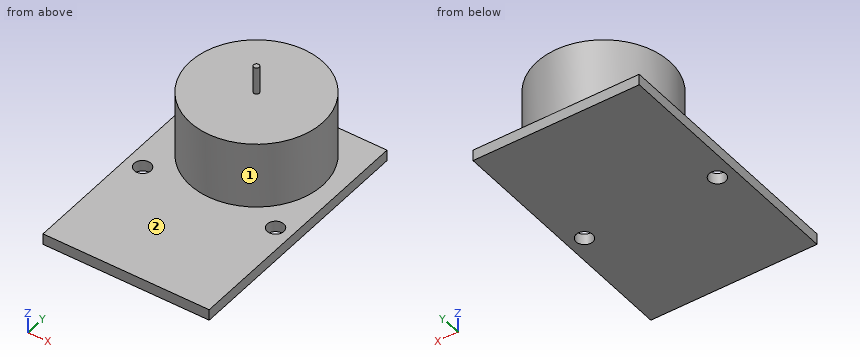
```python
from build123d import *

# Parameters (mm, degrees)
SKETCH_1_W          = 30
SKETCH_1_H          = 45
EXTRUDE_1_DEPTH     = 2
SKETCH_2_R          = 12
EXTRUDE_2_DEPTH     = 12
CUT_EXTRUDE_1_REACH = 31.585
SKETCH_3_R          = 1.5
SKETCH_5_R          = 0.5
EXTRUDE_3_DEPTH     = 5


with BuildPart() as part:
    # 草图1 → 凸台-拉伸1 (new body)
    with BuildSketch(Plane.XY):
        Rectangle(SKETCH_1_W, SKETCH_1_H)
    extrude(amount=-EXTRUDE_1_DEPTH)

    # 草图2 → 凸台-拉伸2 (add)
    with BuildSketch(Plane.XY):
        with Locations(Location((0, 10.5, 0), (0, 0, 90))):
            Circle(SKETCH_2_R)
    extrude(amount=EXTRUDE_2_DEPTH)

    # 草图3 → 切除-拉伸1 (cut, up to next)
    with BuildSketch(Plane.XY, mode=Mode.PRIVATE) as cut_extrude_1_sk1:
        with Locations((-12, -1.5)):
            Circle(SKETCH_3_R)
    cut_extrude_1_tool1 = extrude(cut_extrude_1_sk1.sketch, amount=-CUT_EXTRUDE_1_REACH, mode=Mode.PRIVATE) & part.part
    # 草图3 → 切除-拉伸1 (cut, up to next)
    with BuildSketch(Plane.XY, mode=Mode.PRIVATE) as cut_extrude_1_sk2:
        with Locations(Location((12, -1.5, 0), (0, 0, 180))):
            Circle(SKETCH_3_R)
    cut_extrude_1_tool2 = extrude(cut_extrude_1_sk2.sketch, amount=-CUT_EXTRUDE_1_REACH, mode=Mode.PRIVATE) & part.part
    add(cut_extrude_1_tool1.solids().sort_by_distance((-12, -1.5, 0))[0], mode=Mode.SUBTRACT)
    add(cut_extrude_1_tool2.solids().sort_by_distance((12, -1.5, 0))[0], mode=Mode.SUBTRACT)

    # 草图5 → 凸台-拉伸3 (add)
    with BuildSketch(Plane.XY.offset(12)):
        with Locations((0, 10.5)):
            Circle(SKETCH_5_R)
    extrude(amount=EXTRUDE_3_DEPTH)


solid = part.part
```
Geometry check sheet. Reference: the model listing, model coordinates, mm. Face numbers are marked on the shaded views. Round coordinates to 2 decimals unless told otherwise and drop trailing zeros. Order: outer loops, then holes, each group sorted by start corner. A loop starts at its lowest first (then second) coordinate and runs counter-clockwise, first axis right, second up. Notation, with made-up numbers: (40.25, 73.25) - (86.25, 73.25) arc R28 ccw to (86.25, 100.25) - close; hole circle Ø4 at (-39, 75). An arc over 180 degrees is marked (long way). Use a Markdown table: item, result. Add a question column.
(1) Sectioned sample at B-B, the plane x = -7.75. Enter the section's corners in (y, z), and give its area (3 significant figures).
(2) Release check for a two-part mould opening along Y. For the marked faces 1 and 2 record: pulls with the +Y half, pulls with the -Y half, needs draft (parallel to the pull), parting line crosses it, or undercut.
(3) Sectioned sample at D-D, the plane y = 19. Enter the section's corners in (x, z), and give its area (3 significant figures).
(4) Material ranges on line 1 along Y through (x, z) = (-12, -1); line 2 along Z through (x, y) = (5.75, -20); line 3 along Z through (x, y) = (-3, 10.5), recorded low to high. Write a range as [from, to].
(5) Depth check by flat-ended pin: pin 1 (3.5 mm diameter, centred on x = -12, y = -1.5, fed in from -Z); pin 2 (6 mm diameter, centred on y = 6, z = 10, fed in from -X); pin 3 (4 mm diameter, centred on x = 5, y = 10, fed in from +Z); pin 4 (1 mm diameter, centred on x = -8.5, z = 6, fed in from +Y). Enter the tip coordinate at first touch or a pass-through.
(6) Sectioned sample at C-C, the plane z = 0.5. Enter the section's corners in (x, y), and give its area (3 significant figures).
(7) Sectioned sample at A-A, the plane y = 10.5. Enter the section's corners in (x, z), and give its area (3 significant figures).
Answers below:
| question | item | result |
|---|---|---|
| 1 | outline | (-22.5, -2) - (22.5, -2) - (22.5, 0) - (19.66, 0) - (19.66, 12) - (1.34, 12) - (1.34, 0) - (-22.5, 0) - close |
| 1 | area | 310 mm² |
| 2 | face 1 | parting line crosses it |
| 2 | face 2 | needs draft |
| 3 | outline | (-15, -2) - (15, -2) - (15, 0) - (8.47, 0) - (8.47, 12) - (-8.47, 12) - (-8.47, 0) - (-15, 0) - close |
| 3 | area | 263 mm² |
| 4 | line 1 | [-22.5, -3], [0, 22.5] |
| 4 | line 2 | [-2, 0] |
| 4 | line 3 | [-2, 12] |
| 5 | pin 1 | z = -2 |
| 5 | pin 2 | x = -11.91 |
| 5 | pin 3 | z = 12 |
| 5 | pin 4 | y = 19.44 |
| 6 | outline | circle Ø24 at (0, 10.5) |
| 6 | area | 452 mm² |
| 7 | outline | (-15, -2) - (15, -2) - (15, 0) - (12, 0) - (12, 12) - (0.5, 12) - (0.5, 17) - (-0.5, 17) - (-0.5, 12) - (-12, 12) - (-12, 0) - (-15, 0) - close |
| 7 | area | 353 mm² |
